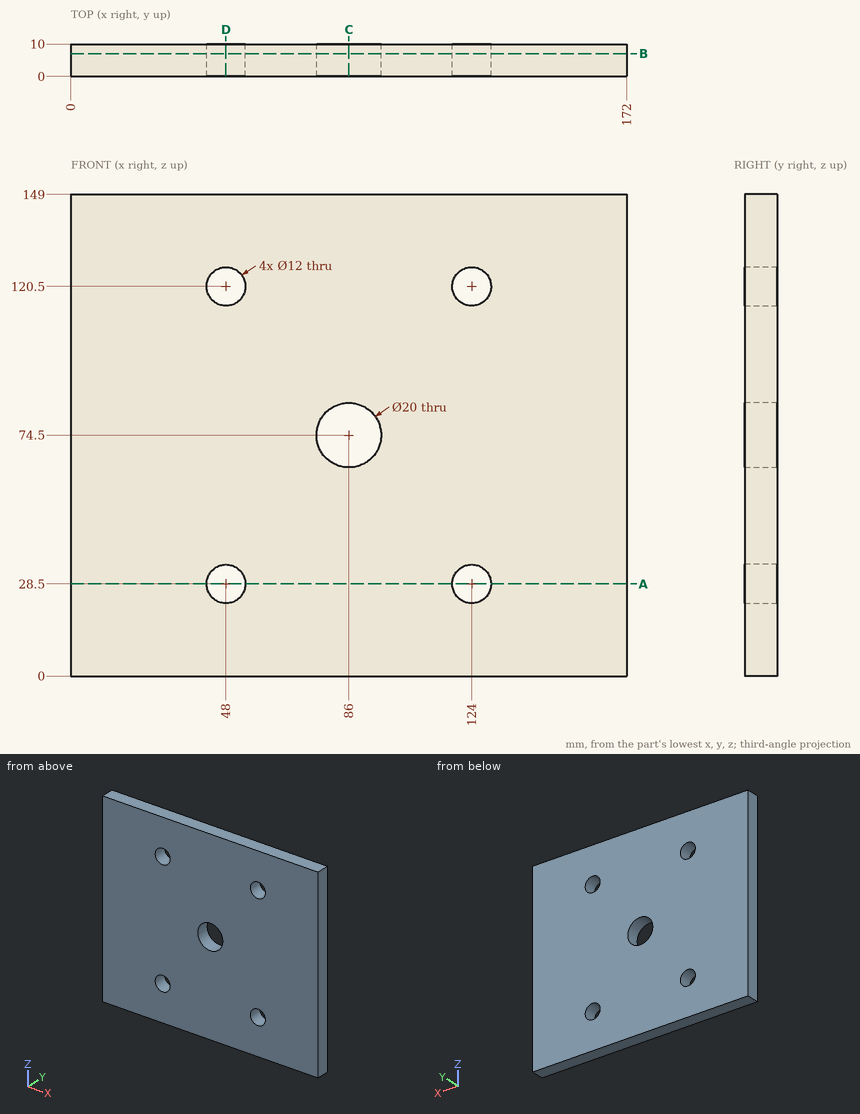
The figure shows three views and two pictorial views of one solid part (mm, origin at its lowest corner). Answer the questions. Coordinates: 2 decimals unless noted, no trailing zeros. Loops run counter-clockwise (first coordinate to the right, second up) from the corner with the lowest first, then second, coordinate; pieces in that order, holes last.
(1) The part is cut by section D-D (x = 48). Determine the outline of the cut face in (y, z).
Solution:
outline: (0, 0) - (10, 0) - (10, 22.5) - (0, 22.5) - close; (0, 34.5) - (10, 34.5) - (10, 114.5) - (0, 114.5) - close; (0, 126.5) - (10, 126.5) - (10, 149) - (0, 149) - close
(2) The part is cut by section C-C (x = 86). Determine the outline of the cut face in (y, z), and give its area (3 significant figures).
Solution:
outline: (0, 0) - (10, 0) - (10, 64.5) - (0, 64.5) - close; (0, 84.5) - (10, 84.5) - (10, 149) - (0, 149) - close
area: 1,290 mm2
(3) Consider line 1 along X through (y, z) = (4.75, 28.5); line 2 along X through (y, z) = (6.25, 25.5); line 3 along Z through (x, y) = (126, 5). Determine where each line is inside the solid, lowest interval first.
Solution:
line 1: x = 0 to 42, 54 to 118, 130 to 172
line 2: x = 0 to 42.8, 53.2 to 118.8, 129.2 to 172
line 3: z = 0 to 22.84, 34.16 to 114.84, 126.16 to 149
(4) The part is cut by section A-A (z = 28.5). Determine the outline of the cut face in (x, y).
Solution:
outline: (0, 0) - (42, 0) - (42, 10) - (0, 10) - close; (54, 0) - (118, 0) - (118, 10) - (54, 10) - close; (130, 0) - (172, 0) - (172, 10) - (130, 10) - close
(5) A flat-ended cylindrical pin translates along its axis: pin 1 Ø15.5 at (x, z) = (124, 120.5) entering from +Y. Find the tip coordinate at first contact, or state that the pin passes through.
Solution:
pin 1: stops at y = 10
(6) The part is cut by section B-B (y = 7). Determine the outline of the cut face in (x, z), and give its area (3 significant figures).
Solution:
outline: (0, 0) - (172, 0) - (172, 149) - (0, 149) - close; hole circle Ø12 at (48, 28.5); hole circle Ø12 at (48, 120.5); hole circle Ø20 at (86, 74.5); hole circle Ø12 at (124, 28.5); hole circle Ø12 at (124, 120.5)
area: 24,900 mm2
